Work out the finished part from the listing and answer in its coordinate system (mm). A direction names the side the tool comes from. Coordinates: 2 decimals unless noted, no trailing zeros. Order: outer loops, then holes, each group sorted by start corner. A loop starts at its lowest first (then second) coordinate and runs counter-clockwise, first axis right, second up.
1. The part is cut by section C-C, the plane z = 2.7. Give the vertices of the cut face in (x, y), then the cut area to 3 significant figures.
2. The part is cut by section A-A, the plane x = 4.25. Give the vertices of the cut face in (y, z), then the cut area to 3 significant figures.
3. The part is cut by section B-B, the plane y = 1.65. Give the vertices of the cut face in (x, z), then the cut area to 3 significant figures.
4. Find the intervals of material crossed by probe 1 along X at (y, z) = (1.4, 2.4); probe 2 along Y at (x, z) = (6.75, 1.65), in increasing order.
5. A tool of negligible diameter and unlimited length cuts with its end or side. For faces 1 (the flat face through (8.08, 1, 2)), 2 (the flat face through (4, 0.5, 2)), from which of +Z, -Z, +X, -X, +Y, -Y can it reach the whole face along a straight path? Write none if from no direction.
6. Determine the mould class of faces 3 (the flat face through (1, 2.5, 2)), 4 (the flat face through (4, 3, 2)), 5 (the flat face through (0, 1, 2)) for opening direction Y: +Y half, -Y half, draft (parallel to the pull), parting line (faces both ways), or undercut.
```python
from build123d import *

# Parameters (mm, degrees)
F0_W     = 8.08
F0_H     = 3
F0_W_2   = 2
F0_H_2   = 2
F1_DEPTH = 5


with BuildPart() as f1:
    # F0 (on Top) → F1 (new body)
    with BuildSketch(Plane.XY):
        with Locations((4.04, 1.5)):
            Rectangle(F0_W, F0_H)
        with Locations((1.5, 1.5)):
            Rectangle(F0_W_2, F0_H_2, mode=Mode.SUBTRACT)
        with Locations((4.04, 1.5)):
            Rectangle(F0_W_2, F0_H_2, mode=Mode.SUBTRACT)
        with Locations((6.58, 1.5)):
            Rectangle(F0_W_2, F0_H_2, mode=Mode.SUBTRACT)
    extrude(amount=F1_DEPTH)


solid = f1.part
```
Geometry says:
1. outline: (0, 0) - (8.08, 0) - (8.08, 3) - (0, 3) - close; hole (0.5, 0.5) - (2.5, 0.5) - (2.5, 2.5) - (0.5, 2.5) - close; hole (3.04, 0.5) - (5.04, 0.5) - (5.04, 2.5) - (3.04, 2.5) - close; hole (5.58, 0.5) - (7.58, 0.5) - (7.58, 2.5) - (5.58, 2.5) - close
1. area: 12.2 mm2
2. outline: (0, 0) - (0.5, 0) - (0.5, 5) - (0, 5) - close; (2.5, 0) - (3, 0) - (3, 5) - (2.5, 5) - close
2. area: 5.00 mm2
3. outline: (0, 0) - (0.5, 0) - (0.5, 5) - (0, 5) - close; (2.5, 0) - (3.04, 0) - (3.04, 5) - (2.5, 5) - close; (5.04, 0) - (5.58, 0) - (5.58, 5) - (5.04, 5) - close; (7.58, 0) - (8.08, 0) - (8.08, 5) - (7.58, 5) - close
3. area: 10.4 mm2
4. probe 1: x = 0 to 0.5, 2.5 to 3.04, 5.04 to 5.58, 7.58 to 8.08
4. probe 2: y = 0 to 0.5, 2.5 to 3
5. face 1: +Z, -Z, +X, +Y, -Y
5. face 2: +Z, -Z
6. face 3: undercut
6. face 4: +Y half
6. face 5: draft
